Here's how the part is built. I have some questions about the finished solid (model axes, mm). A direction names the side the tool comes from. Round coordinates to 2 decimals unless told otherwise and drop trailing zeros. Order: outer loops, then holes, each group sorted by start corner. A loop starts at its lowest first (then second) coordinate and runs counter-clockwise, first axis right, second up. Notation, with made-up numbers: (66.5, -26.5) - (110.5, -26.5) arc R24 ccw to (110.5, -11.5) - close; hole circle Ø7 at (37.5, 46). An arc over 180 degrees is marked (long way). One line per item, written item: value.
Autodesk Inventor part; units mm, degrees
ref_plane "YZ Plane" through (0, 0, 0) normal (1, 0, 0) x (0, 1, 0)
ref_plane "XZ Plane" through (0, 0, 0) normal (0, 1, 0) x (-1, 0, 0)
ref_plane "XY Plane" through (0, 0, 0) normal (0, 0, 1) x (1, 0, 0)
sketch "Sketch1" plane through (0, 0, 0) normal (0, 1, 0) x (-1, 0, 0)
  arc A0 (-159.7794, 702.6597) -> (-160.5669, 701.8721) centre (-159.7794, 701.8721) ccw
  line L0 (-159.7794, 702.6597) -> (-155.7462, 702.6597)
  line L1 (-155.7462, 702.6597) -> (-155.7462, 704.2667)
  line L2 (-155.7462, 704.2667) -> (-153.4941, 704.2667)
  line L3 (-153.4941, 704.2667) -> (-153.4941, 703.5159)
  line L4 (-153.4941, 703.5159) -> (-152.5972, 703.5159)
  arc A1 (-164.1836, 648.4268) -> (-160.5669, 657.8731) centre (-174.7114, 657.8731) ccw
  line L5 (-160.5669, 657.8731) -> (-160.5669, 701.8721)
  arc A2 (-160.1794, 645.8656) -> (-160.7583, 645.6139) centre (-160.1783, 645.0714) ccw
  arc A3 (-164.1836, 648.4268) -> (-160.7583, 645.6139) centre (-162.4137, 647.0901) ccw
  line L6 (-160.1794, 645.8656) -> (-155.7462, 645.8656)
  line L7 (-155.7462, 645.8656) -> (-155.7462, 644.2582)
  line L8 (-155.7462, 644.2582) -> (-153.4959, 644.2582)
  line L9 (-153.4959, 644.2582) -> (-153.4959, 645.3298)
  line L10 (-153.4959, 645.3298) -> (-152.5301, 645.3298)
  line L11 (-152.5301, 645.3298) -> (-142.8493, 642.7649)
  arc A4 (-143.0499, 641.0266) -> (-142.8493, 642.7649) centre (-143.1468, 641.9185) ccw
  line L12 (-163.0475, 641.9081) -> (-143.0499, 641.0266)
  arc A5 (-166.5264, 650.2868) -> (-163.0475, 641.9081) centre (-162.4021, 647.0877) ccw
  arc A6 (-166.5264, 650.2868) -> (-167.6429, 666.7468) centre (-174.8334, 657.9912) ccw
  line L13 (-167.6429, 666.7468) -> (-167.6429, 671.3153)
  arc A7 (-166.8471, 672.1213) -> (-167.6429, 671.3153) centre (-166.8257, 671.3043) ccw
  line L14 (-166.8471, 672.1213) -> (-166.0512, 672.1176)
  arc A8 (-165.304, 671.5825) -> (-166.0512, 672.1176) centre (-166.0579, 671.319) ccw
  line L15 (-165.304, 671.5825) -> (-164.5204, 669.4361)
  line L16 (-164.5204, 669.4361) -> (-164.4882, 669.3468)
  arc A9 (-164.4882, 669.3468) -> (-164.2374, 669.1723) centre (-164.2343, 669.4443) ccw
  line L17 (-164.2374, 669.1723) -> (-163.8302, 669.1723)
  arc A10 (-163.8326, 669.1723) -> (-163.5671, 669.4384) centre (-163.8364, 669.4416) ccw
  line L18 (-163.5671, 669.4384) -> (-163.5671, 706.0242)
  line L19 (-163.5671, 706.0242) -> (-163.5671, 706.0613)
  line L20 (-163.5671, 706.0613) -> (-147.5434, 708.8923)
  arc A11 (-147.5434, 708.8923) -> (-147.8025, 710.4755) centre (-147.5845, 709.6983) ccw
  line L21 (-147.8025, 710.4755) -> (-163.5671, 707.6952)
  line L22 (-163.5671, 707.6952) -> (-164.9603, 707.6952)
  line L23 (-164.9603, 707.6952) -> (-164.9605, 706.5472)
  arc A12 (-165.374, 706.3282) -> (-164.9605, 706.5472) centre (-165.23, 706.5562) ccw
  line L24 (-165.374, 706.3282) -> (-167.226, 707.3966)
  arc A13 (-167.6397, 708.1008) -> (-167.226, 707.3966) centre (-166.8384, 708.0979) ccw
  line L25 (-167.6397, 708.1008) -> (-167.6393, 713.6964)
  arc A14 (-166.8357, 714.5011) -> (-167.6393, 713.6964) centre (-166.8345, 713.6963) ccw
  line L26 (-166.8357, 714.5011) -> (-164.1567, 714.5011)
  arc A15 (-163.353, 713.6974) -> (-164.1567, 714.5011) centre (-164.1583, 713.6958) ccw
  line L27 (-163.353, 713.6974) -> (-163.353, 712.3579)
  line L28 (-163.353, 712.3579) -> (-165.4962, 711.98)
  line L29 (-165.4962, 711.98) -> (-165.4962, 711.7118)
  arc A16 (-165.4962, 711.7118) -> (-163.8213, 710.1096) centre (-163.8924, 711.7118) ccw
  line L30 (-163.8213, 710.1096) -> (-146.2918, 713.1784)
  arc A17 (-144.5878, 707.1017) -> (-146.2918, 713.1784) centre (-146.018, 709.9779) ccw
  line L31 (-144.5878, 707.1017) -> (-152.2275, 703.608)
  arc A18 (-152.5972, 703.5159) -> (-152.2275, 703.608) centre (-152.6033, 704.3289) ccw
  point P0 (-160.5669, 683.588)
  dimension "d1" = 90
  dimension "d2" = 43.999
  dimension "d3" = 3.0002
extrude "Extrusion1" add sketch "Sketch1" along normal blind 5.3
properties part number "raspDinClipmmv1"
Q1. If we section it at D-D, the plane z = 668.5: Please give me the cut outline in (x, y).
Results list:
outline: (160.57, 0) - (167.64, 0) - (167.64, 5.3) - (160.57, 5.3) - close
Q2. Which directions (+Z, -Z, +X, -X, +Y, -Y) give clear straight access to the entire face, cutting with the end or side of a thin tool? Please do faces 4 (the flat face through (167.643, 3, 669)), 5 (the flat face through (166.287, 2.613, 706.855)), 6 (the flat face through (163.353, 3, 713)), 7 (the flat face through (155.746, 3, 703)), 8 (the flat face through (147.757, 2.613, 644.065)).
Results list:
face 4: +Z, -Z, +X, +Y, -Y
face 5: +X, +Y, -Y
face 6: +Z, +Y, -Y
face 7: +Y, -Y
face 8: -X, +Y, -Y
Q3. If we section it at C-C, the plane x = 155: Please give me the cut outline in (y, z), then the cut area to 3 significant figures.
Results list:
outline: (0, 641.55) - (5.3, 641.55) - (5.3, 644.26) - (0, 644.26) - close; (0, 704.27) - (5.3, 704.27) - (5.3, 707.57) - (0, 707.57) - close; (0, 709.21) - (5.3, 709.21) - (5.3, 711.65) - (0, 711.65) - close
area: 44.8 mm²
Q4. If we section it at B-B, the plane z = 681: Please give me the cut outline in (x, y), then the cut area to 3 significant figures.
Results list:
outline: (160.57, 0) - (163.57, 0) - (163.57, 5.3) - (160.57, 5.3) - close
area: 15.9 mm²
Q5. We'd pull the mould along X, two halves only. Please class faces 1 (the flat face through (153.189, 2.613, 641.474)), 2 (the flat face through (148.35, 2.61, 705.38)), 3 (the flat face through (155.746, 3, 645)): released by +X, released by -X, zero draft, split by the parting line, or undercut.
Results list:
face 1: released by +X
face 2: released by -X
face 3: undercut
Q6. If I drill on line 1 along Z through (x, y) = (150.5, 0.8) (3 decimals); line 2 along Z through (x, y) = (166, 4.35); line 3 along X through (y, z) = (3.8, 703), over which ranges is the centre line in solid material (lowest first)?
Results list:
line 1: 641.355 to 644.792, 704.398 to 708.37, 710 to 712.442
line 2: 643.31 to 650.9, 665.09 to 672.12, 706.69 to 714.5
line 3: 155.75 to 163.57
Q7. If we section it at A-A, the plane x = 161.75: Please give me the cut outline in (y, z).
Results list:
outline: (0, 641.85) - (5.3, 641.85) - (5.3, 644.97) - (0, 644.97) - close; (0, 652.21) - (5.3, 652.21) - (5.3, 706.38) - (0, 706.38) - close; (0, 708.02) - (5.3, 708.02) - (5.3, 710.47) - (0, 710.47) - close
Q8. Will these pins go through, and if not, where does the flat tip stop? pin 1 (2 mm diameter, centred on x = 157, y = 4, fed in from -Z); pin 2 (1.1 mm diameter, centred on y = 2.5, z = 713, fed in from -X); pin 3 (1 mm diameter, centred on y = 1.5, z = 659.5, fed in from -X); pin 4 (1.5 mm diameter, centred on x = 147.58, z = 709.7, fed in from -Y).
Results list:
pin 1: z = 641.6
pin 2: x = 143.97
pin 3: x = 160.57
pin 4: through
